Verification items for the finished model (mm, model axes). A direction names the side the tool comes from. Round coordinates to 2 decimals unless told otherwise and drop trailing zeros. Loops run counter-clockwise (first coordinate to the right, second up) from the corner with the lowest first, then second, coordinate; pieces in that order, holes last. Notation, with made-up numbers: M 17.25,22.25 L 50.25,22.25 A14 ccw 50.25,30.25 Z; hole C 62.25,-27.75 d1. An arc over 180 degrees is marked long. One line per item, written item: value.
Autodesk Inventor part; units mm, degrees
ref_plane "YZ Plane" through (0, 0, 0) normal (1, 0, 0) x (0, 1, 0)
ref_plane "XZ Plane" through (0, 0, 0) normal (0, 1, 0) x (-1, 0, 0)
ref_plane "XY Plane" through (0, 0, 0) normal (0, 0, 1) x (1, 0, 0)
sketch "Sketch1" plane through (0, 0, 0) normal (0, 0, 1) x (1, 0, 0)
  line L0 (104.168, 1.684) -> (742.0066, 617.6375)
  arc A0 (100, 0) -> (104.168, 1.684) centre (100, 6) ccw
  line L1 (0, 0) -> (100, 0)
  dimension "d25" = 6
  dimension "d48" = 742.0065
  dimension "d49" = 136
  dimension "d50" = 100
  dimension "d51" = 886.7
contour flange "Contour Flange1" sketch "Sketch1" thickness 3 bend radius 3 width 980 along (0, 0, 1) mid plane no both sides no wall seen from (50, 0, 0) lies toward (0, 1, 0) curves L1 A0 L0
bend "Bend1"
corner "Corner1"
mirror "Mirror1" about plane through (0, 0, 0) normal (1, 0, 0)
sketch "Sketch2" plane through (-102.084, 3.842, 980) normal (0.6946584, 0.7193398, 0) x (0.7193398, -0.6946584, 0)
  line L0 (-842.2117, 70.9383) -> (-842.2117, 209.5784) construction
  line L1 (-842.2117, 209.5784) -> (-819.3515, 209.5784) construction
  line L2 (-819.3515, 209.5784) -> (-819.3515, 70.9383) construction
  line L3 (-819.3515, 70.9383) -> (-842.2117, 70.9383) construction
  point P0 (76.1019, 980)
mark "Mark1"
equation "\"d25\" = Thickness + BendRadius"
equation "\"d7\" = Thickness"
equation "\"d8\" = BendReliefWidth"
equation "\"d9\" = BendReliefDepth"
equation "\"d10\" = MinimumRemnant"
equation "\"d11\" = TransitionRadius"
equation "\"d13\" = BendRadius"
equation "\"d15\" = CornerReliefSize"
equation "\"d16\" = GapSize"
equation "\"d17\" = JacobiRadiusSize"
equation "\"BendRadius\" = Thickness"
equation "\"BendReliefWidth\" = Thickness"
equation "\"BendReliefDepth\" = 0.5 * Thickness"
equation "\"CornerReliefSize\" = 4 * Thickness"
equation "\"MinimumRemnant\" = 2 * Thickness"
equation "\"TransitionRadius\" = BendRadius"
equation "\"JacobiRadiusSize\" = BendRadius"
equation "\"GapSize\" = Thickness"
equation "\"d38\" = d40 + d44"
equation "\"d39\" = d40"
equation "\"d44\" = d40"
properties part number "MSC 501 SHEET BELLY MAIN" material "Stainless Steel"
(1) Mould release check, pull along X, two halves, no side actions. Record for faces 1 (the face through (416.54, 307.51, 483.14)), 2 (the face through (-427.55, 313.97, 483.14)), 3 (the face through (-1, 0, 483)): +X half, -X half, draft (parallel to the pull), parting line (faces both ways), or undercut.
Completed:
face 1: undercut
face 2: -X half
face 3: draft
(2) Depth check by flat-ended pin: pin 1 Ø6 at (x, y) = (-243.5, 128.5) entering from -Z; pin 2 Ø5 at (y, z) = (324, 243) entering from -X; pin 3 Ø10 at (x, z) = (481.5, 547) entering from -Y; pin 4 Ø2 at (x, z) = (-399, 148) entering from -Y. Enter the tip coordinate at first touch or a pass-through.
Completed:
pin 1: passes through
pin 2: stops at x = -440.52
pin 3: stops at y = 361.24
pin 4: stops at y = 285.43
(3) Thickness scan on L1, parallel to X at y = 208, z = 366; L2, parallel to X at y = 201, z = 708.5; L3, parallel to Y at x = -407, z = 900. Record the ranges inside material, lowest first. Write a range as from..to.
Completed:
L1: x = -317.81..-313.5, 313.5..317.81
L2: x = -310.57..-306.25, 306.25..310.57
L3: y = 294.13..298.3
(4) Sectioned sample at B-B on z = 616. Enter the section's corners in (x, y), and give its area (3 significant figures).
Completed:
outline: M -742.01,617.64 L -104.17,1.68 A6 ccw -100,0 L 100,0 A6 ccw 104.17,1.68 L 742.01,617.64 L 739.92,619.8 L 102.08,3.84 A3 cw 100,3 L -100,3 A3 cw -102.08,3.84 L -739.92,619.8 Z
area: 5,940 mm^2
(5) Sectioned sample at D-D on x = 178.5. Enter the section's corners in (y, z).
Completed:
outline: M 73.47,0 L 77.64,0 L 77.64,980 L 73.47,980 Z
(6) Sectioned sample at A-A on y = 509.5. Enter the section's corners in (x, z), and give its area (3 significant figures).
Completed:
outline: M -630.03,0 L -625.71,0 L -625.71,980 L -630.03,980 Z; M 625.71,0 L 630.03,0 L 630.03,980 L 625.71,980 Z
area: 8,460 mm^2
(7) Tool access check on faces 4 (the face through (-1, 3, 483)), 5 (the face through (418.622, 305.349, 483.14)). Record the directions out of +Z, -Z, +X, -X, +Y, -Y that give a thin tool (end or side, any length) a straight path to the whole face; none if there is none.
Completed:
face 4: +Z, -Z, +Y
face 5: +Z, -Z, +X, -Y
(8) Sectioned sample at C-C on x = -4. Enter the section's corners in (y, z), and give its area (3 significant figures).
Completed:
outline: M 0,0 L 3,0 L 3,980 L 0,980 Z
area: 2,940 mm^2
